Geometry: final body of the model. Coordinates: model frame, mm. A direction names the side the tool comes from. Coordinates: 2 decimals unless noted, no trailing zeros. Write each loop counter-clockwise with the first axis right and the second up, starting at its lowest first coordinate (ties: lowest second). Pieces come first, ordered by that corner, then holes. Notation, with made-up numbers: (-29.75, 32) - (5.25, 32) arc R19 cw to (5.25, 53) - close; hole circle Ø10 at (-20, 28.25). An arc over 180 degrees is marked (long way). Answer as a JSON object with one key per item and string values. Group by question number.
Item 1: Section A-A on x = 3. Return loops of the section in (y, z), and give its area (3 significant figures).
Item 2: Line query: line 1 along Z through (x, y) = (-29, -33.5); line 2 along X through (y, z) = (-17.5, 5); line 3 along Z through (x, y) = (18, -40). Output: solid intervals per line, ascending. Write a range as from..to.
Item 3: Section B-B on z = -11.5. Return loops of the section in (x, y).
Item 4: First-contact query: pin 1 Ø3 at (y, z) = (-32, 9.5) entering from -X; pin 2 Ø4 at (x, y) = (30, -38) entering from +Z; pin 3 Ø2 at (y, z) = (-17, 4.5) entering from -X; pin 4 Ø3 at (x, z) = (-30.5, -24) entering from -Y. Flat tips, straight axial feed; report the tip coordinate or a pass-through.
Item 5: Set-up query: faces 1 (the cylindrical face through (-29.31, -25.04, 16.09)), 2 (the cylindrical face through (-28.49, -25.04, -17.5)), 3 (the flat face through (14.42, -25, 34)), 4 (the flat face through (-21.1, -25, -30.3)), 5 (the flat face through (37, -25, 0)). Return all of +Z, -Z, +X, -X, +Y, -Y with unobstructed straight access to the full face (end or side cutting, diameter ignored); none if empty.
Item 6: Mould query, pull axis Z, two halves, no side actions, for faces 6 (the flat face through (-14.49, -25.04, 37.45)), 7 (the flat face through (-37, -25, 3.256)), 8 (the cylindrical face through (4.685, -25.044, -33.107)). Classes: pulls with the +Z half, pulls with the -Z half, needs draft (parallel to the pull), parting line crosses it, or undercut.
```python
from build123d import *

# Parameters (mm, degrees)
F0_R     = 19.61617
F1_DEPTH = 50.8


with BuildPart() as f1:
    # F0 (on Front) → F1 (new body)
    with BuildSketch(Plane.XZ):
        with BuildLine():
            Line((-6.052636, 39.878492), (-6.052636, 32.884275))
            ThreePointArc((-6.052636, 32.884275), (-7.548644, 32.573424), (-9.028888, 32.194551))
            Line((-9.028888, 32.194551), (-11.007963, 38.804037))
            Line((-11.007963, 38.804037), (-18.076009, 36.058098))
            Line((-18.076009, 36.058098), (-14.738214, 30.013247))
            ThreePointArc((-14.738214, 30.013247), (-17.441313, 28.527365), (-19.995981, 26.798707))
            Line((-19.995981, 26.798707), (-25.037277, 31.623777))
            Line((-25.037277, 31.623777), (-32.690295, 23.627805))
            Line((-32.690295, 23.627805), (-27.349421, 19.235881))
            ThreePointArc((-27.349421, 19.235881), (-29.333744, 16.048096), (-30.948132, 12.657925))
            Line((-30.948132, 12.657925), (-38.297591, 12.657925))
            Line((-38.297591, 12.657925), (-40.203536, 3.256409))
            Line((-40.203536, 3.256409), (-33.277707, 3.256409))
            ThreePointArc((-33.277707, 3.256409), (-33.413831, -1.235271), (-32.946427, -5.704638))
            Line((-32.946427, -5.704638), (-39.573435, -7.802038))
            Line((-39.573435, -7.802038), (-36.856234, -16.387391))
            Line((-36.856234, -16.387391), (-30.628721, -13.41236))
            ThreePointArc((-30.628721, -13.41236), (-28.455593, -17.558165), (-25.724808, -21.359874))
            Line((-25.724808, -21.359874), (-29.741899, -27.246063))
            ThreePointArc((-29.741899, -27.246063), (-26.367109, -30.523829), (-22.633617, -33.386343))
            Line((-22.633617, -33.386343), (-19.527745, -27.141797))
            ThreePointArc((-19.527745, -27.141797), (-15.172234, -29.796196), (-10.463662, -31.757231))
            Line((-10.463662, -31.757231), (-10.463662, -38.954336))
            ThreePointArc((-10.463662, -38.954336), (-5.277192, -39.988496), (0, -40.335202))
            Line((0, -40.335202), (0, -33.436656))
            ThreePointArc((0, -33.436656), (4.750751, -33.097437), (9.405108, -32.086663))
            Line((9.405108, -32.086663), (12.953476, -38.198639))
            ThreePointArc((12.953476, -38.198639), (17.318161, -36.428147), (21.446691, -34.160913))
            Line((21.446691, -34.160913), (18.053638, -28.143847))
            ThreePointArc((18.053638, -28.143847), (21.60412, -25.52003), (24.777977, -22.451321))
            Line((24.777977, -22.451321), (30.581673, -26.299997))
            ThreePointArc((30.581673, -26.299997), (33.096887, -23.054818), (35.269166, -19.570756))
            Line((35.269166, -19.570756), (29.892103, -14.982395))
            ThreePointArc((29.892103, -14.982395), (31.173038, -12.093454), (32.175517, -9.096488))
            Line((32.175517, -9.096488), (39.296087, -9.096488))
            Line((39.296087, -9.096488), (40.335202, 0))
            Line((40.335202, 0), (33.436656, 0))
            ThreePointArc((33.436656, 0), (33.177826, 4.152331), (32.405342, 8.240376))
            Line((32.405342, 8.240376), (38.766721, 11.138667))
            Line((38.766721, 11.138667), (34.556119, 20.803923))
            Line((34.556119, 20.803923), (28.816288, 16.959703))
            Line((28.816288, 16.959703), (24.398983, 22.862625))
            Line((24.398983, 22.862625), (25.948878, 30.88016))
            Line((25.948878, 30.88016), (14.420494, 37.669323))
            Line((14.420494, 37.669323), (14.420494, 30.167189))
            ThreePointArc((14.420494, 30.167189), (10.326321, 31.802155), (6.052636, 32.884275))
            Line((6.052636, 32.884275), (6.052636, 39.878492))
            ThreePointArc((6.052636, 39.878492), (0, 40.335202), (-6.052636, 39.878492))
        make_face()
        Circle(F0_R, mode=Mode.SUBTRACT)
    extrude(amount=F1_DEPTH)


solid = f1.part
```
Checks:
{
 "1": {"outline": "(-50.8, -33.3) - (0, -33.3) - (0, -19.39) - (-50.8, -19.39) - close; (-50.8, 19.39) - (0, 19.39) - (0, 40.22) - (-50.8, 40.22) - close", "area": "1,770 mm^2"},
 "2": {"line 1": "-28.03..-26.16, -16.64..16.64, 20.59..27.48", "line 2": "-39.85..-18.97, 18.97..33.06", "line 3": "-36.1..-7.8, 7.8..35.56"},
 "3": {"outline": "(-38.4, -50.8) - (-15.89, -50.8) - (-15.89, 0) - (-38.4, 0) - close; (15.89, -50.8) - (31.4, -50.8) - (31.4, 0) - (15.89, 0) - close"},
 "4": {"pin 1": "x = -39.24", "pin 2": "z = 19.09", "pin 3": "x = -40.15", "pin 4": "through"},
 "5": {"face 1": "-X, +Y, -Y", "face 2": "+Y, -Y", "face 3": "+Z, +Y, -Y", "face 4": "-Z, +Y, -Y", "face 5": "+X, +Y, -Y"},
 "6": {"face 6": "pulls with the +Z half", "face 7": "undercut", "face 8": "pulls with the -Z half"}
}
